Check sheet for the drawn part. Datum: minimum x, y, z corner. Units: mm. A direction names the side the tool comes from. Give positions to 0.01 mm unless a question says otherwise; leave off trailing zeros. Loops run counter-clockwise (first coordinate to the right, second up) from the corner with the lowest first, then second, coordinate; pieces in that order, holes last. Notation, with made-up numbers: (32.25, 29) - (58.25, 29) arc R30 cw to (58.25, 68) - close; hole circle Ø6 at (13, 43.25). An arc over 180 degrees is marked (long way). Use a Markdown table: item, result. Add a question column.
1. Cross-section at C-C on z = 7.5. Enter the section's corners in (x, y).
2. Draft check along Y on the marked faces 6, 7 and 8. Enter one of: pulls with the +Y half, pulls with the -Y half, needs draft (parallel to the pull), parting line crosses it, or undercut.
3. Set-up check for the marked faces 1, 2, 3, 4 and 5: record each of +Z, -Z, +X, -X, +Y, -Y from which the full face is reachable in a straight line by a thin tool's end or side.
4. Depth check by flat-ended pin: P1, Ø5.5, axis at y = 3.5, z = 7.5, coming from the -X side; P2, Ø0.9, axis at x = 1.5, y = 8, coming from the -Z side; P3, Ø2.5, axis at x = 1.5, z = 26, coming from the +Y side; P4, Ø2.5, axis at x = 2, y = 9, coming from the +Z side. Enter the tip coordinate at first touch or a pass-through.
5. Cross-section at A-A on x = 1.25. Enter the section's corners in (y, z).
6. Material ranges on L1, parallel to Y at x = 3.1, z = 22.5; L2, parallel to Y at x = 0.9, z = 22.5; L3, parallel to Z at x = 1.65, y = 9, recorded low to high.
7. Cross-section at B-B on y = 3.5. Enter the section's corners in (x, z), and give its area (3 significant figures).
8. Cross-section at D-D on x = 2.5. Enter the section's corners in (y, z), and give its area (3 significant figures).
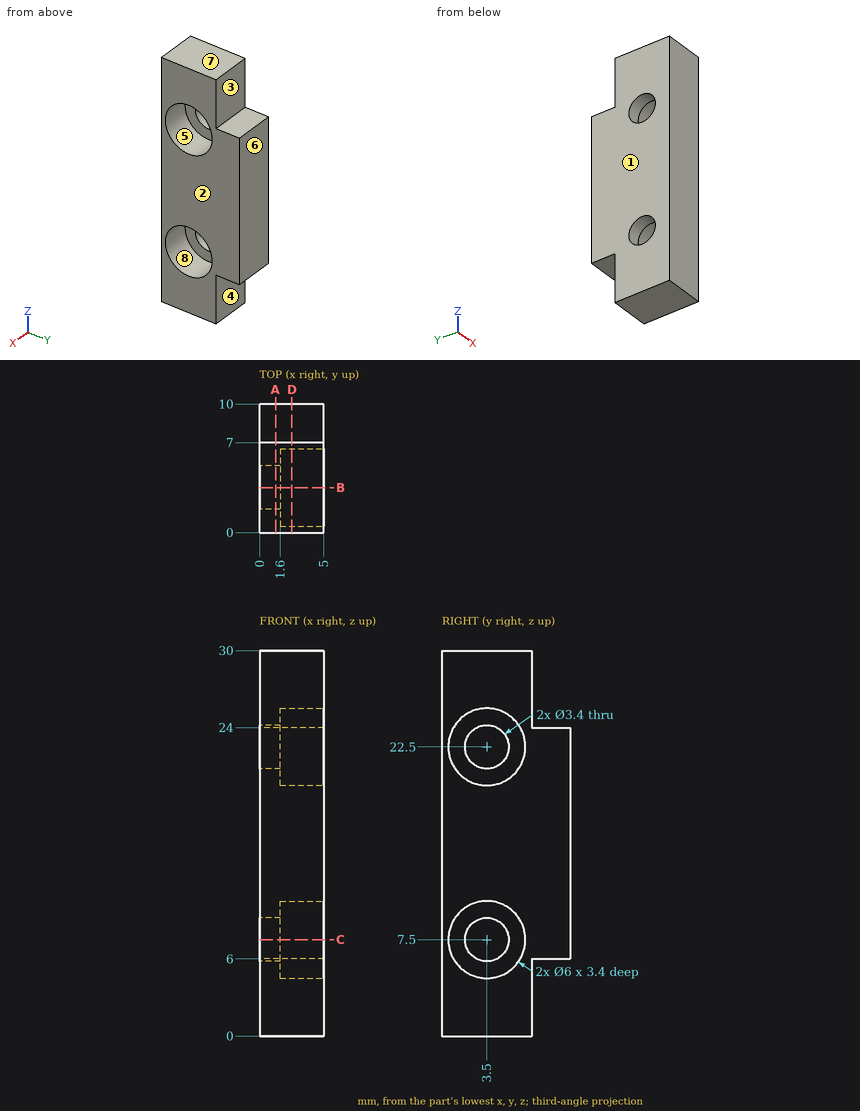
Values found:
| question | item | result |
|---|---|---|
| 1 | outline | (0, 0) - (5, 0) - (5, 0.5) - (1.6, 0.5) - (1.6, 1.8) - (0, 1.8) - close; (0, 5.2) - (1.6, 5.2) - (1.6, 6.5) - (5, 6.5) - (5, 10) - (0, 10) - close |
| 2 | face 6 | pulls with the +Y half |
| 2 | face 7 | needs draft |
| 2 | face 8 | undercut |
| 3 | face 1 | +Z, -Z, -X, +Y, -Y |
| 3 | face 2 | +Z, -Z, +X, +Y, -Y |
| 3 | face 3 | +Z, +X, -X, +Y |
| 3 | face 4 | -Z, +X, -X, +Y |
| 3 | face 5 | +X |
| 4 | P1 | stops at x = 0 |
| 4 | P2 | stops at z = 6 |
| 4 | P3 | stops at y = 7 |
| 4 | P4 | stops at z = 24 |
| 5 | outline | (0, 0) - (7, 0) - (7, 6) - (10, 6) - (10, 24) - (7, 24) - (7, 30) - (0, 30) - close; hole circle Ø3.4 at (3.5, 7.5); hole circle Ø3.4 at (3.5, 22.5) |
| 6 | L1 | y = 0 to 0.5, 6.5 to 10 |
| 6 | L2 | y = 0 to 1.8, 5.2 to 10 |
| 6 | L3 | z = 6 to 24 |
| 7 | outline | (0, 0) - (5, 0) - (5, 4.5) - (1.6, 4.5) - (1.6, 5.8) - (0, 5.8) - close; (0, 9.2) - (1.6, 9.2) - (1.6, 10.5) - (5, 10.5) - (5, 19.5) - (1.6, 19.5) - (1.6, 20.8) - (0, 20.8) - close; (0, 24.2) - (1.6, 24.2) - (1.6, 25.5) - (5, 25.5) - (5, 30) - (0, 30) - close |
| 7 | area | 98.3 mm2 |
| 8 | outline | (0, 0) - (7, 0) - (7, 6) - (10, 6) - (10, 24) - (7, 24) - (7, 30) - (0, 30) - close; hole circle Ø6 at (3.5, 7.5); hole circle Ø6 at (3.5, 22.5) |
| 8 | area | 207 mm2 |
